```python
from build123d import *


with BuildPart() as part:
    # Sketch1 → Revolve1 (revolve)
    with BuildSketch(Plane.XY):
        with BuildLine():
            Line((0, 71.4), (0, 0))
            Line((0, 0), (5, 0))
            Line((5, 0), (6, 1))
            Line((6, 1), (6, 35))
            Line((6, 35), (7.5, 35))
            Line((7.5, 35), (7.5, 56.8))
            Line((7.5, 56.8), (6, 56.8))
            Line((6, 56.8), (6, 67.3))
            Line((6, 67.3), (5.75, 67.3))
            Line((5.75, 67.3), (5.75, 68.4))
            Line((5.75, 68.4), (6, 68.4))
            Line((6, 68.4), (6, 69.4))
            ThreePointArc((6, 69.4), (5.414213562, 70.814213562), (4, 71.4))
            Line((4, 71.4), (0, 71.4))
        make_face()
    revolve(axis=Axis((0, 71.4, 0), (0, -1, 0)))


solid = part.part
```
The model under review builds one solid part; all positions refer to its coordinate system, in mm. A direction names the side the tool comes from. Round coordinates to 2 decimals unless told otherwise and drop trailing zeros. Order: outer loops, then holes, each group sorted by start corner. A loop starts at its lowest first (then second) coordinate and runs counter-clockwise, first axis right, second up. Notation, with made-up numbers: (71, -16) -> (86, -16) arc R18 ccw to (86, -12) -> close; hole circle Ø6 at (11.5, 30). An arc over 180 degrees is marked (long way). One line per item, written item: value. Start each with the question number.
Q1. Wall thickness on line 1 (X direction, y = 26, z = -0.25); line 2 (Y direction, x = 2, z = 6.5); line 3 (X direction, y = 40.5, z = -5.75): over which ranges is each line inside the solid? List them lowest first.
Q2. Take a section at B-B (z = 0). Write out the cut boundary in (x, y), and give its area (3 significant figures).
Q3. Take a section at A-A (x = 0). Write out the cut boundary in (y, z), and give its area (3 significant figures).
Q4. Mouldability with a two-part tool opening along Y and no side actions: class faces 4 (the face through (-0.75, 67.86, 5.7)), 5 (the face through (-6, 62, 0)), 6 (the face through (-2, 35, 6)) as released by +Y, released by -Y, zero draft, split by the parting line, or undercut.
Q5. Clearance check with flat-ended pins moving along their axes: pin 1 Ø1 at (x, z) = (-4, 5.5) entering from -Y; pin 2 Ø5 at (x, y) = (1, 31) entering from -Z; pin 3 Ø2 at (x, z) = (4, -6) entering from +Y. State where each tip first meets the part, or that it passes through.
Q6. Machinability: for faces 1 (the face through (-7.493, 46.053, 0.33)), 2 (the face through (-6, 18, 0)), 3 (the face through (-6, 69, 0)), which of the approach directions +Z, -Z, +X, -X, +Y, -Y give a long, thin tool a straight path to every point of the face, cutting with its end or side? Answer none if there is none.
Q7. Take a section at D-D (y = 22). Write out the cut boundary in (x, z), and give its area (3 significant figures).
Q8. Take a section at C-C (y = 47). Write out the cut boundary in (x, z).
Reported:
1. line 1: x = -5.99 to 5.99
1. line 2: y = 35 to 56.8
1. line 3: x = -4.82 to 4.82
2. outline: (-7.5, 35) -> (-6, 35) -> (-6, 1) -> (-5, 0) -> (5, 0) -> (6, 1) -> (6, 35) -> (7.5, 35) -> (7.5, 56.8) -> (6, 56.8) -> (6, 67.3) -> (5.75, 67.3) -> (5.75, 68.4) -> (6, 68.4) -> (6, 69.4) arc R2 ccw to (4, 71.4) -> (-4, 71.4) arc R2 ccw to (-6, 69.4) -> (-6, 68.4) -> (-5.75, 68.4) -> (-5.75, 67.3) -> (-6, 67.3) -> (-6, 56.8) -> (-7.5, 56.8) -> close
2. area: 919 mm2
3. outline: (0, -5) -> (1, -6) -> (35, -6) -> (35, -7.5) -> (56.8, -7.5) -> (56.8, -6) -> (67.3, -6) -> (67.3, -5.75) -> (68.4, -5.75) -> (68.4, -6) -> (69.4, -6) arc R2 ccw to (71.4, -4) -> (71.4, 4) arc R2 ccw to (69.4, 6) -> (68.4, 6) -> (68.4, 5.75) -> (67.3, 5.75) -> (67.3, 6) -> (56.8, 6) -> (56.8, 7.5) -> (35, 7.5) -> (35, 6) -> (1, 6) -> (0, 5) -> close
3. area: 919 mm2
4. face 4: undercut
4. face 5: zero draft
4. face 6: released by -Y
5. pin 1: stops at y = 35
5. pin 2: stops at z = -6
5. pin 3: stops at y = 56.8
6. face 1: +Y, -Y
6. face 2: -Y
6. face 3: +Y
7. outline: circle Ø12 at (0, 0)
7. area: 113 mm2
8. outline: circle Ø15 at (0, 0)
